Study the drawing (mm; zero at the part's minimum x, y, z) and answer. A direction names the side the tool comes from. Give positions to 0.01 mm unless a question says otherwise; leave off trailing zeros. Write each loop counter-clockwise with the first axis right and the second up, starting at its lowest first coordinate (ties: lowest second). Pieces come first, ordered by that corner, then holes.
1) Find section C-C (y = 17). Determine the outline of the cut face in (x, z), plus the area to 3 significant figures.
2) Given pin 1 Ø4 at (y, z) = (30.5, 5) entering from -X; pin 2 Ø7.5 at (y, z) = (7.5, 12) entering from +X; pin 3 Ø5 at (x, z) = (49, 12.5) entering from -Y, each flat-ended and moving along its own axis, determine where each tip first touches the part or whether it passes through.
3) A tool of negligible diameter and unlimited length cuts with its end or side. For the marked faces 1, 2, 3, 4 and 5, from which of +Z, -Z, +X, -X, +Y, -Y can it reach the whole face along a straight path? Write none if from no direction.
4) Find section B-B (x = 16.7). Determine the outline of the cut face in (y, z).
5) Find section D-D (z = 18.5). Determine the outline of the cut face in (x, y).
6) Find section A-A (z = 10). Determine the outline of the cut face in (x, y).
7) Straight lines are drawn through the part: probe 1 along Y at (x, z) = (16.5, 19); probe 2 along X at (y, z) = (40, 13.5); probe 3 along Y at (x, z) = (48.5, 1). For each, find the intervals that lie inside material, in ascending order.
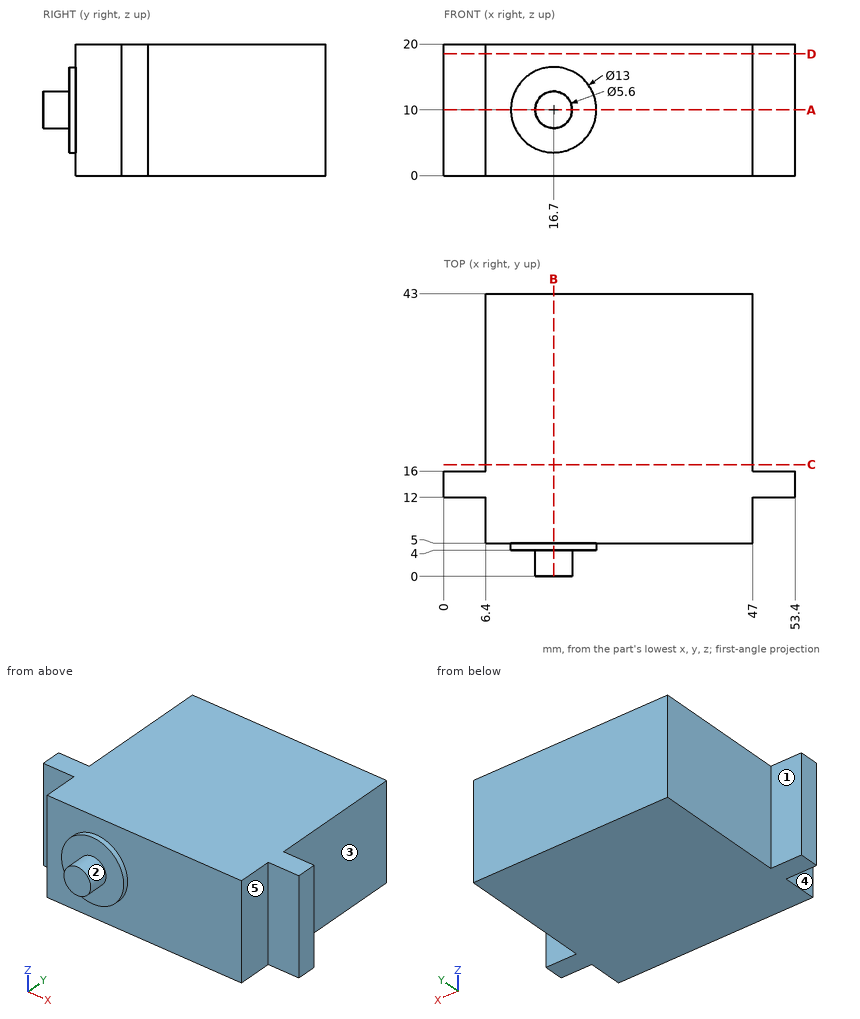
Results:
1. outline: (6.4, 0) - (47, 0) - (47, 20) - (6.4, 20) - close
1. area: 812 mm2
2. pin 1: stops at x = 6.4
2. pin 2: stops at x = 47
2. pin 3: stops at y = 5
3. face 1: +Z, -Z, -X, +Y
3. face 2: -Y
3. face 3: +Z, -Z, +X, +Y
3. face 4: +Z, -Z, -X, -Y
3. face 5: +Z, -Z, +X, -Y
4. outline: (0, 7.2) - (4, 7.2) - (4, 3.5) - (5, 3.5) - (5, 0) - (43, 0) - (43, 20) - (5, 20) - (5, 16.5) - (4, 16.5) - (4, 12.8) - (0, 12.8) - close
5. outline: (0, 12) - (6.4, 12) - (6.4, 5) - (47, 5) - (47, 12) - (53.4, 12) - (53.4, 16) - (47, 16) - (47, 43) - (6.4, 43) - (6.4, 16) - (0, 16) - close
6. outline: (0, 12) - (6.4, 12) - (6.4, 5) - (10.2, 5) - (10.2, 4) - (13.9, 4) - (13.9, 0) - (19.5, 0) - (19.5, 4) - (23.2, 4) - (23.2, 5) - (47, 5) - (47, 12) - (53.4, 12) - (53.4, 16) - (47, 16) - (47, 43) - (6.4, 43) - (6.4, 16) - (0, 16) - close
7. probe 1: y = 5 to 43
7. probe 2: x = 6.4 to 47
7. probe 3: y = 12 to 16
